from build123d import *

# Parameters (mm, degrees)
F1_DEPTH  = 2
F2_W      = 2
F2_H      = 190
F3_DEPTH  = 53
F4_R      = 1
F5_W      = 10
F5_H      = 186
F6_DEPTH  = 2
F7_R      = 1
F8_W      = 224
F8_H      = 2
F9_DEPTH  = 9
F10_R     = 1
F11_W     = 0.5
F11_H     = 1
F12_DEPTH = 235.001
F13_R     = 7.5
F14_DEPTH = 3
F15_R     = 1.2
F16_DEPTH = 3
F17_R     = 1.2
F18_DEPTH = 190.001
F19_W     = 120
F19_H     = 20
F20_DEPTH = 3


with BuildPart() as f1:
    # F0 (on Top) → F1 (new body)
    with BuildSketch(Plane.XY):
        Polygon((112.5, -95), (117.5, -95), (117.5, 95), (112.5, 95), (112.5, 92), (112, 92), (112, 95), (-112, 95), (-112, 92), (-112.5, 92), (-112.5, 95), (-117.5, 95), (-117.5, -95), (-112.5, -95), (-112.5, -92), (-112, -92), (-112, -95), (112, -95), (112, -92), (112.5, -92), align=None)
    extrude(amount=F1_DEPTH)

    # F2 (on face) → F3 (join)
    with BuildSketch(Plane.XY.offset(2)):
        with Locations((116.5, 0)):
            Rectangle(F2_W, F2_H)
        with Locations((-116.5, 0)):
            Rectangle(F2_W, F2_H)
    extrude(amount=F3_DEPTH)

    # F4
    f4_edges = [f1.edges().sort_by_distance(p)[0] for p in [
        (-117.5, 0, 0),
        (117.5, 0, 0),
        (-115.5, 0, 2),
        (115.5, 0, 2),
    ]]
    fillet(f4_edges, radius=F4_R)

    # F5 (on face) → F6 (join)
    with BuildSketch(Plane.XY.offset(55)):
        with Locations((-112.5, 0)):
            Rectangle(F5_W, F5_H)
        with Locations((112.5, 0)):
            Rectangle(F5_W, F5_H)
    extrude(amount=F6_DEPTH)

    # F7
    f7_edges = [f1.edges().sort_by_distance(p)[0] for p in [
        (-117.5, 0, 57),
        (117.5, 0, 57),
        (-115.5, 0, 55),
        (115.5, 0, 55),
    ]]
    fillet(f7_edges, radius=F7_R)

    # F8 (on face) → F9 (join)
    with BuildSketch(Plane.XY.offset(2)):
        with Locations((0, -94)):
            Rectangle(F8_W, F8_H)
        with Locations((0, 94)):
            Rectangle(F8_W, F8_H)
    extrude(amount=F9_DEPTH)

    # F10
    f10_edges = [f1.edges().sort_by_distance(p)[0] for p in [
        (0, -95, 0),
        (0, -93, 2),
        (0, 93, 2),
        (0, 95, 0),
    ]]
    fillet(f10_edges, radius=F10_R)

    # F11 (on face) → F12 (cut, through all)
    with BuildSketch(Plane(origin=(-117.5, 0, 0), x_dir=(0, -1, 0), z_dir=(-1, 0, 0))):
        with Locations((93.25, 54.5)):
            Rectangle(F11_W, F11_H)
        with Locations((-93.25, 54.5)):
            Rectangle(F11_W, F11_H)
    extrude(amount=-F12_DEPTH, mode=Mode.SUBTRACT)

    # F13 (on face) → F14 (cut)
    with BuildSketch(Plane(origin=(-117.5, 0, 0), x_dir=(0, -1, 0), z_dir=(-1, 0, 0))):
        with Locations((63, 30)):
            Circle(F13_R)
    extrude(amount=-F14_DEPTH, mode=Mode.SUBTRACT)

    # F15 (on face) → F16 (cut)
    with BuildSketch(Plane.XY.offset(2)):
        with Locations((-109.5, 87)):
            Circle(F15_R)
        with Locations((109.5, 87)):
            Circle(F15_R)
        with Locations((-109.5, -87)):
            Circle(F15_R)
        with Locations((109.5, -87)):
            Circle(F15_R)
        with Locations((-21.5, 60)):
            Circle(F15_R)
        with Locations((73.5, 60)):
            Circle(F15_R)
        with Locations((-21.5, -60)):
            Circle(F15_R)
        with Locations((73.5, -60)):
            Circle(F15_R)
        with Locations((-45.5, 17)):
            Circle(F15_R)
        with Locations((-45.5, -23)):
            Circle(F15_R)
        with Locations((-45.5, -63)):
            Circle(F15_R)
    extrude(amount=-F16_DEPTH, mode=Mode.SUBTRACT)

    # F17 (on face) → F18 (cut, through all)
    with BuildSketch(Plane.XZ.offset(95)):
        with Locations((104, 7)):
            Circle(F17_R)
        with Locations((-104, 7)):
            Circle(F17_R)
    extrude(amount=-F18_DEPTH, mode=Mode.SUBTRACT)

    # F19 (on face) → F20 (cut)
    with BuildSketch(Plane.YZ.offset(117.5)):
        with Locations((0, 17)):
            Rectangle(F19_W, F19_H)
    extrude(amount=-F20_DEPTH, mode=Mode.SUBTRACT)


solid = f1.part
Here's how the part is built. I have some questions about the finished solid (model axes, mm). A direction names the side the tool comes from. Coordinates: 2 decimals unless noted, no trailing zeros. Order: outer loops, then holes, each group sorted by start corner. A loop starts at its lowest first (then second) coordinate and runs counter-clockwise, first axis right, second up. Notation, with made-up numbers: (79.5, -4.75) -> (115.5, -4.75) arc R24 ccw to (115.5, 23.25) -> close; hole circle Ø11 at (46.5, 75.5). An arc over 180 degrees is marked (long way). Answer in a Markdown table with one row per item.
(1) Will these pins go through, and if not, where does the flat tip stop? pin 1 Ø1.4 at (x, y) = (109.5, -87) entering from -Z; pin 2 Ø1.2 at (x, y) = (-116, -94) entering from +Z; pin 3 Ø1.4 at (x, y) = (-45.5, 17) entering from -Z; pin 4 Ø3.5 at (x, z) = (-112, 55.5) entering from +Y.
Answer key:
| item | result |
|---|---|
| pin 1 | z = 55 |
| pin 2 | z = 55 |
| pin 3 | through |
| pin 4 | y = 93 |
(2) I want a section at B-B on y = -11. List the corners of the cut face in (x, z) for me.
Answer key:
| item | result |
|---|---|
| outline | (-117.5, 1) arc R1 ccw to (-116.5, 0) -> (116.5, 0) arc R1 ccw to (117.5, 1) -> (117.5, 7) -> (115.5, 7) -> (115.5, 3) arc R1 cw to (114.5, 2) -> (-114.5, 2) arc R1 cw to (-115.5, 3) -> (-115.5, 54) arc R1 cw to (-114.5, 55) -> (-107.5, 55) -> (-107.5, 57) -> (-116.5, 57) arc R1 ccw to (-117.5, 56) -> close; (107.5, 55) -> (114.5, 55) arc R1 cw to (115.5, 54) -> (115.5, 27) -> (117.5, 27) -> (117.5, 56) arc R1 ccw to (116.5, 57) -> (107.5, 57) -> close |
(3) Please list where these lines run through material, in increasing order: probe 1 along X at (y, z) = (87, 1.05); probe 2 along Y at (x, z) = (109.5, 1.1); probe 3 along X at (y, z) = (62, 8).
Answer key:
| item | result |
|---|---|
| probe 1 | -117.5 to -110.7, -108.3 to 108.3, 110.7 to 117.5 |
| probe 2 | -95 to -88.2, -85.8 to 85.8, 88.2 to 95 |
| probe 3 | -117.5 to -115.5, 115.5 to 117.5 |
(4) I want a section at C-C on x = 98.5. List the corners of the cut face in (y, z) for me, then the cut area to 3 significant figures.
Answer key:
| item | result |
|---|---|
| outline | (-95, 1) arc R1 ccw to (-94, 0) -> (94, 0) arc R1 ccw to (95, 1) -> (95, 11) -> (93, 11) -> (93, 3) arc R1 cw to (92, 2) -> (-92, 2) arc R1 cw to (-93, 3) -> (-93, 11) -> (-95, 11) -> close |
| area | 416 mm^2 |
(5) I want a section at D-D on y = 75. List the corners of the cut face in (x, z) for me, then the cut area to 3 significant figures.
Answer key:
| item | result |
|---|---|
| outline | (-117.5, 1) arc R1 ccw to (-116.5, 0) -> (116.5, 0) arc R1 ccw to (117.5, 1) -> (117.5, 56) arc R1 ccw to (116.5, 57) -> (107.5, 57) -> (107.5, 55) -> (114.5, 55) arc R1 cw to (115.5, 54) -> (115.5, 3) arc R1 cw to (114.5, 2) -> (-114.5, 2) arc R1 cw to (-115.5, 3) -> (-115.5, 54) arc R1 cw to (-114.5, 55) -> (-107.5, 55) -> (-107.5, 57) -> (-116.5, 57) arc R1 ccw to (-117.5, 56) -> close |
| area | 722 mm^2 |
(6) Thinking about a two-plate mould opening in Z: for faces 1 (the face through (-112, 1, 57)), 2 (the face through (117.5, -1, 28)), 3 (the face through (111, 1, 55)), which applies, +Z half, -Z half, draft (parallel to the pull), parting line (faces both ways), or undercut?
Answer key:
| item | result |
|---|---|
| face 1 | +Z half |
| face 2 | draft |
| face 3 | undercut |
(7) On a 3-axis mill with a long thin cutter (end or side, diameter ignored), from which of +Z, -Z, +X, -X, +Y, -Y can I reach the whole of each face in a straight line? I mean faces 4 (the face through (-111, 1, 55)), 5 (the face through (-116, 95, 27)), 6 (the face through (-116.51, -61.37, 22.68)). Say none if no direction works.
Answer key:
| item | result |
|---|---|
| face 4 | +Y, -Y |
| face 5 | +Z, -Z, +X, -X, +Y |
| face 6 | -X |
(8) I want a section at A-A on z = 47. List the corners of the cut face in (x, y) for me, then the cut area to 3 significant figures.
Answer key:
| item | result |
|---|---|
| outline | (-117.5, -95) -> (-115.5, -95) -> (-115.5, 95) -> (-117.5, 95) -> close; (115.5, -95) -> (117.5, -95) -> (117.5, 95) -> (115.5, 95) -> close |
| area | 760 mm^2 |
